The drawing under review shows one solid part. Ordinate dimensions are in mm from its lowest x, y, z. Coordinates: 2 decimals unless noted, no trailing zeros. Order: outer loops, then holes, each group sorted by start corner. A loop starts at its lowest first (then second) coordinate and runs counter-clockwise, first axis right, second up. Notation, with made-up numbers: (40, 42) -> (87, 42) arc R14 cw to (87, 52) -> close; hole circle Ø9 at (40, 31.25). An arc over 180 degrees is marked (long way). Put each result on its own line as item: value.
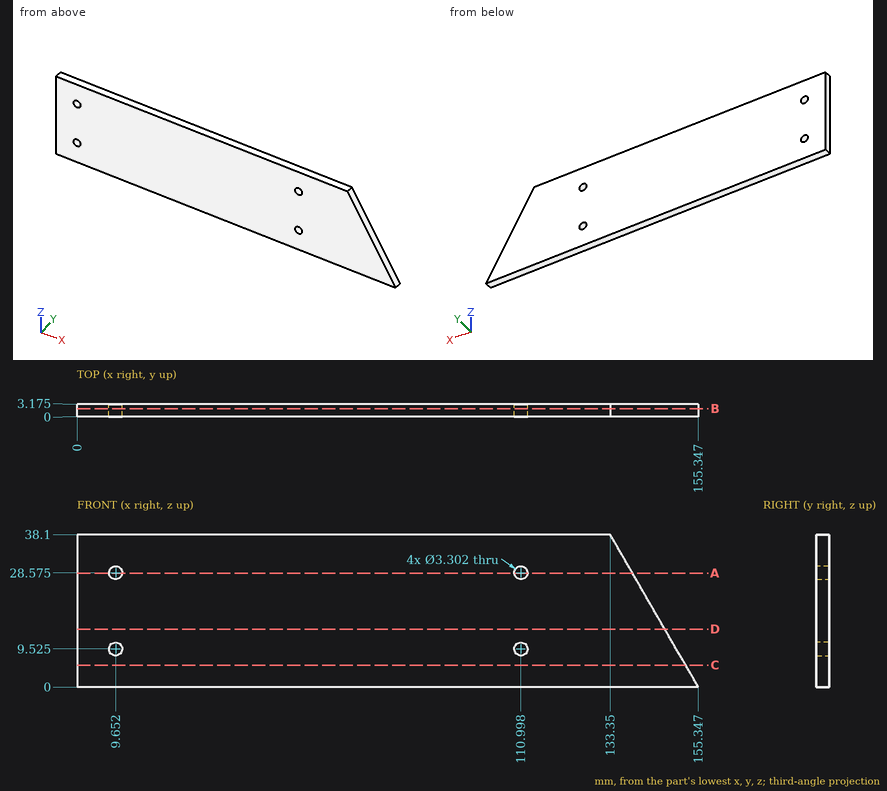
Item 1: Consider section D-D on z = 14.5. Write out the cut boundary in (x, y) (1 decimal), and give its area (3 significant figures).
Answers below:
outline: (0, 0) -> (147, 0) -> (147, 3.2) -> (0, 3.2) -> close
area: 467 mm^2
Item 2: Consider section B-B on y = 2. Write out the cut boundary in (x, z) (3 decimals).
Answers below:
outline: (0, 0) -> (155.347, 0) -> (133.35, 38.1) -> (0, 38.1) -> close; hole circle Ø3.302 at (9.652, 9.525); hole circle Ø3.302 at (9.652, 28.575); hole circle Ø3.302 at (110.998, 9.525); hole circle Ø3.302 at (110.998, 28.575)
Item 3: For line 1 (X direction, y = 0.6, z = 8.5); line 2 (Z direction, x = 112, y = 2.35); line 3 (X direction, y = 0.75, z = 10), list the stretches that pass through material, from the lowest coordinate up. Write a range as from..to.
Answers below:
line 1: 0..8.36, 10.95..109.7, 112.29..150.44
line 2: 0..8.21, 10.84..27.26, 29.89..38.1
line 3: 0..8.07, 11.23..109.42, 112.58..149.57
Item 4: For pin 1 Ø3 at (x, z) = (9.652, 28.575) entering from -Y, flat-tipped, find the tip position at first contact; note if it passes through.
Answers below:
pin 1: through
Item 5: Consider section C-C on z = 5.5. Write out the cut boundary in (x, y) (3 decimals), and give its area (3 significant figures).
Answers below:
outline: (0, 0) -> (152.172, 0) -> (152.172, 3.175) -> (0, 3.175) -> close
area: 483 mm^2
Item 6: Consider section A-A on z = 28.5. Write out the cut boundary in (x, y) (1 decimal).
Answers below:
outline: (0, 0) -> (8, 0) -> (8, 3.2) -> (0, 3.2) -> close; (11.3, 0) -> (109.3, 0) -> (109.3, 3.2) -> (11.3, 3.2) -> close; (112.6, 0) -> (138.9, 0) -> (138.9, 3.2) -> (112.6, 3.2) -> close
